```python
from build123d import *

# Parameters (mm, degrees)
F0_W     = 8.333958
F0_H     = 95.447298
F0_W_2   = 6.184932
F1_DEPTH = 25.4
F2_DEPTH = 50.8
F3_R     = 2.54


with BuildPart() as f1:
    # F0 (on Top) → F1 (new body)
    with BuildSketch(Plane.XY):
        with Locations((-43.55667, 0)):
            Rectangle(F0_W, F0_H)
        with Locations((43.55667, 0)):
            Rectangle(F0_W, F0_H)
        with Locations((36.297225, 0)):
            Rectangle(F0_W_2, F0_H)
        with Locations((21.778335, 0)):
            Rectangle(F0_W_2, F0_H)
        with Locations((7.259445, 0)):
            Rectangle(F0_W_2, F0_H)
        with Locations((-7.259445, 0)):
            Rectangle(F0_W_2, F0_H)
        with Locations((-21.778335, 0)):
            Rectangle(F0_W_2, F0_H)
        with Locations((-36.297225, 0)):
            Rectangle(F0_W_2, F0_H)
        with Locations((-29.03778, 0)):
            Rectangle(F0_W, F0_H)
        with Locations((-14.51889, 0)):
            Rectangle(F0_W, F0_H)
        Rectangle(F0_W, F0_H)
        with Locations((14.51889, 0)):
            Rectangle(F0_W, F0_H)
        with Locations((29.03778, 0)):
            Rectangle(F0_W, F0_H)
    extrude(amount=-F1_DEPTH)

    # F0 (on Top) → F2 (join)
    with BuildSketch(Plane.XY):
        with Locations((-43.55667, 0)):
            Rectangle(F0_W, F0_H)
        with Locations((-29.03778, 0)):
            Rectangle(F0_W, F0_H)
        with Locations((-14.51889, 0)):
            Rectangle(F0_W, F0_H)
        Rectangle(F0_W, F0_H)
        with Locations((14.51889, 0)):
            Rectangle(F0_W, F0_H)
        with Locations((29.03778, 0)):
            Rectangle(F0_W, F0_H)
        with Locations((43.55667, 0)):
            Rectangle(F0_W, F0_H)
    extrude(amount=F2_DEPTH)

    # F3
    f3_edges = [f1.edges().sort_by_distance(p)[0] for p in [
        (-47.723649, 0, 50.8),
        (-39.389691, 0, 50.8),
        (-33.204759, 0, 50.8),
        (-24.870801, 0, 50.8),
        (-18.685869, 0, 50.8),
        (-10.351911, 0, 50.8),
        (-4.166979, 0, 50.8),
        (4.166979, 0, 50.8),
        (10.351911, 0, 50.8),
        (18.685869, 0, 50.8),
        (24.870801, 0, 50.8),
        (33.204759, 0, 50.8),
        (39.389691, 0, 50.8),
        (47.723649, 0, 50.8),
        (33.204759, 0, 0),
        (18.685869, 0, 0),
        (4.166979, 0, 0),
        (-10.351911, 0, 0),
        (-24.870801, 0, 0),
        (-39.389691, 0, 0),
        (-33.204759, 0, 0),
        (-18.685869, 0, 0),
        (-4.166979, 0, 0),
        (10.351911, 0, 0),
        (24.870801, 0, 0),
        (39.389691, 0, 0),
    ]]
    fillet(f3_edges, radius=F3_R)


solid = f1.part
```
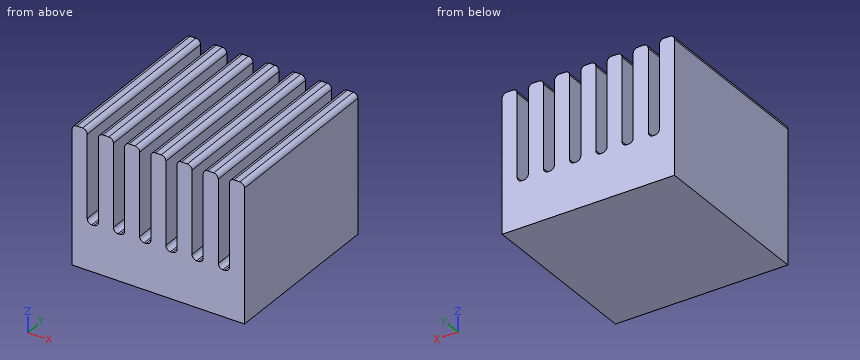
CAD build for the part. Positions are in the model's coordinates, mm. Round coordinates to 2 decimals unless told otherwise and drop trailing zeros. Order: outer loops, then holes, each group sorted by start corner. A loop starts at its lowest first (then second) coordinate and runs counter-clockwise, first axis right, second up. Notation, with made-up numbers: (-7.75, 82) - (13.25, 82) arc R29 ccw to (13.25, 118) - close; hole circle Ø8 at (29.25, 70.5). An arc over 180 degrees is marked (long way). Answer as CSV lines item,"result". Start each with the question number.
1. Pin check, flat tip, straight feed: pin 1 (1.5 mm diameter, centred on x = -36.5, y = -37.5, fed in from +Z). Stop position of the tip, or through.
2. Saw through at A-A, the plane z = 7.5. Write the cut outline in (x, y), and give its area (3 significant figures).
3. Drill centre lines: L1, parallel to Z at x = -7.5, y = -40; L2, parallel to Z at x = -24, y = -1. Where is each one in solid material? Low to high. Write a range as [from, to].
Model answer:
1,pin 1,"stops at z = 0.03"
2,outline,"(-47.72, -47.72) - (-39.39, -47.72) - (-39.39, 47.72) - (-47.72, 47.72) - close; (-33.2, -47.72) - (-24.87, -47.72) - (-24.87, 47.72) - (-33.2, 47.72) - close; (-18.69, -47.72) - (-10.35, -47.72) - (-10.35, 47.72) - (-18.69, 47.72) - close; (-4.17, -47.72) - (4.17, -47.72) - (4.17, 47.72) - (-4.17, 47.72) - close; (10.35, -47.72) - (18.69, -47.72) - (18.69, 47.72) - (10.35, 47.72) - close; (24.87, -47.72) - (33.2, -47.72) - (33.2, 47.72) - (24.87, 47.72) - close; (39.39, -47.72) - (47.72, -47.72) - (47.72, 47.72) - (39.39, 47.72) - close"
2,area,"5,570 mm²"
3,L1,"z = [-25.4, 0]"
3,L2,"z = [-25.4, 0.63]"
